Verification items for the finished model (mm, model axes). A direction names the side the tool comes from. Coordinates: 2 decimals unless noted, no trailing zeros. Write each loop counter-clockwise with the first axis right and the second up, starting at its lowest first coordinate (ties: lowest second). Pieces come first, ordered by that corner, then holes. Notation, with made-up numbers: M 78,7.5 L 136,7.5 A8 cw 136,15.5 Z; hole C 63,21 d6. An arc over 180 degrees is marked long. One line per item, written item: value.
```python
from build123d import *

# Parameters (mm, degrees)
CROQUIS1_R                 = 6
SALIENTE_EXTRUIR1_DEPTH    = 10
CROQUIS2_R                 = 4
SALIENTE_EXTRUIR2_DEPTH    = 10
CROQUIS3_R                 = 4.25
CORTAR_EXTRUIR1_DEPTH      = 8
CROQUIS4_R                 = 2
CORTAR_EXTRUIR2_DEPTH      = 7
CORTAR_EXTRUIR2_DEPTH_BACK = 7


with BuildPart() as part:
    # Croquis1 → Saliente-Extruir1 (new body)
    with BuildSketch(Plane(origin=(0, 0, 0), x_dir=(1, 0, 0), z_dir=(0, 1, 0))):
        Circle(CROQUIS1_R)
    extrude(amount=SALIENTE_EXTRUIR1_DEPTH)

    # Croquis2 → Saliente-Extruir2 (add)
    with BuildSketch(Plane(origin=(0, 10, 0), x_dir=(1, 0, 0), z_dir=(0, 1, 0))):
        Circle(CROQUIS2_R)
    extrude(amount=SALIENTE_EXTRUIR2_DEPTH)

    # Croquis3 → Cortar-Extruir1 (cut)
    with BuildSketch(Plane.XZ):
        Circle(CROQUIS3_R)
    extrude(amount=-CORTAR_EXTRUIR1_DEPTH, mode=Mode.SUBTRACT)

    # Croquis4 → Cortar-Extruir2 (cut, two sides)
    with BuildSketch(Plane.XY) as cortar_extruir2_sk:
        with Locations((0, 4)):
            Circle(CROQUIS4_R)
    extrude(amount=CORTAR_EXTRUIR2_DEPTH, mode=Mode.SUBTRACT)
    extrude(cortar_extruir2_sk.sketch, amount=-CORTAR_EXTRUIR2_DEPTH_BACK, mode=Mode.SUBTRACT)


solid = part.part
```
Item 1: Cross-section at D-D, the plane y = 12.25. Enter the section's corners in (x, z), and give its area (3 significant figures).
The answers:
outline: C 0,0 d8
area: 50.3 mm²
Item 2: Draft check along Z on faces 1 (the face through (-0.867, 14.93, 3.905)), 2 (the face through (3.926, 3.944, -1.628)), 3 (the face through (3, 0, 4)). Enter one of: released by +Z, released by -Z, zero draft, split by the parting line, or undercut.
The answers:
face 1: split by the parting line
face 2: undercut
face 3: zero draft
Item 3: Cross-section at C-C, the plane x = 2.5. Enter the section's corners in (y, z).
The answers:
outline: M 0,-5.45 L 10,-5.45 L 10,-3.12 L 20,-3.12 L 20,3.12 L 10,3.12 L 10,5.45 L 0,5.45 L 0,3.44 L 8,3.44 L 8,-3.44 L 0,-3.44 Z
Item 4: Cross-section at A-A, the plane z = 0. Enter the section's corners in (x, y).
The answers:
outline: M -6,0 L -4.25,0 L -4.25,8 L 4.25,8 L 4.25,0 L 6,0 L 6,10 L 4,10 L 4,20 L -4,20 L -4,10 L -6,10 Z
Item 5: Access from +Z, -Z, +X, -X, +Y, -Y to the whole of each face (thin tool, end or side, straight path). Record for faces 4 (the face through (1.847, 3.234, -4.86)), 5 (the face through (-1.42, 10, 3.92)), 6 (the face through (0, 8, 0)).
The answers:
face 4: +Z, -Z
face 5: +Y
face 6: -Y
Item 6: Go/stop test with flat-tipped pins: P1, Ø2, axis at y = 8, z = 1.5, coming from the -X side; P2, Ø2, axis at y = 14, z = -2.5, coming from the +X side; P3, Ø4, axis at x = -2, y = 15, coming from the -Z side; P4, Ø3, axis at x = 0, y = 4, coming from the +Z side. Record where each tip stops, or that it passes through.
The answers:
P1: stops at x = -5.98
P2: stops at x = 3.71
P3: stops at z = -4
P4: passes through
Item 7: Cross-section at B-B, the plane y = 3.5. Enter the section's corners in (x, z), and give its area (3 significant figures).
The answers:
outline: M -1.94,-5.68 L -1.94,-3.78 A4.25 cw -1.94,3.78 L -1.94,5.68 A6 ccw Z; M 1.94,-5.68 A6 ccw 1.94,5.68 L 1.94,3.78 A4.25 cw 1.94,-3.78 Z
area: 42.4 mm²
Item 8: Scan lines: line 1 (Y direction, x = 0, z = 4.35); line 2 (Y direction, x = 2.75, z = -2.25); line 3 (Y direction, x = -4.5, z = -2). Record each from-to range of solid material in increasing order.
The answers:
line 1: y = 0 to 2, 6 to 10
line 2: y = 8 to 20
line 3: y = 0 to 10
